Here's how the part is built. I have some questions about the finished solid (model axes, mm). A direction names the side the tool comes from. Round coordinates to 2 decimals unless told otherwise and drop trailing zeros. Loops run counter-clockwise (first coordinate to the right, second up) from the corner with the lowest first, then second, coordinate; pieces in that order, holes last. Notation, with made-up numbers: M 75.5,36.25 L 88.5,36.25 A14 cw 88.5,61.25 Z; hole C -7.75,49 d5. An arc over 180 degrees is marked long. Answer as CSV lines item,"result".
```python
from build123d import *

# Parameters (mm, degrees)
ESQUISSE1_R             = 15
BOSS_EXTRU_1_DEPTH      = 10
ESQUISSE5_R             = 6.75
ESQUISSE5_R_2           = 172
ENL_V_MAT_EXTRU_1_DEPTH = 10
CONG_1_R                = 40
ENL_V_MAT_EXTRU_2_DEPTH = 10


with BuildPart() as part:
    # Esquisse1 → Boss.-Extru.1 (new body)
    with BuildSketch(Plane(origin=(0, 0, 0), x_dir=(0, 0, -1), z_dir=(1, 0, 0))):
        Polygon((540, 0), (540, 340), (195, 340), (0, 180), (0, 0), (0, -100), (540, -100), align=None)
        with Locations((490, 300)):
            Circle(ESQUISSE1_R, mode=Mode.SUBTRACT)
        with Locations((50, 160)):
            Circle(ESQUISSE1_R, mode=Mode.SUBTRACT)
    extrude(amount=BOSS_EXTRU_1_DEPTH)

    # Esquisse5 → Enlèv. mat.-Extru.1 (cut)
    with BuildSketch(Plane.ZY):
        with Locations((-270, 325)):
            Circle(ESQUISSE5_R)
        with Locations((-217.389629624, 317.768871033)):
            Circle(ESQUISSE5_R)
        with Locations((-270, 130)):
            Circle(ESQUISSE5_R_2)
        with Locations((-168.681129743, 296.611783887)):
            Circle(ESQUISSE5_R)
        with Locations((-127.486986966, 263.097862928)):
            Circle(ESQUISSE5_R)
        with Locations((-96.862382412, 219.712682358)):
            Circle(ESQUISSE5_R)
        with Locations((-79.078602902, 169.673922545)):
            Circle(ESQUISSE5_R)
        with Locations((-75.454590008, 116.692729394)):
            Circle(ESQUISSE5_R)
        with Locations((-86.259120187, 64.698475627)):
            Circle(ESQUISSE5_R)
        with Locations((-110.690870863, 17.547337188)):
            Circle(ESQUISSE5_R)
        with Locations((-146.937850856, -21.263701687)):
            Circle(ESQUISSE5_R)
        with Locations((-192.31178748, -48.856203794)):
            Circle(ESQUISSE5_R)
        with Locations((-243.447503426, -63.183759477)):
            Circle(ESQUISSE5_R)
        with Locations((-296.552496574, -63.183759477)):
            Circle(ESQUISSE5_R)
        with Locations((-347.68821252, -48.856203794)):
            Circle(ESQUISSE5_R)
        with Locations((-393.062149144, -21.263701687)):
            Circle(ESQUISSE5_R)
        with Locations((-429.309129137, 17.547337188)):
            Circle(ESQUISSE5_R)
        with Locations((-453.740879813, 64.698475627)):
            Circle(ESQUISSE5_R)
        with Locations((-464.545409992, 116.692729394)):
            Circle(ESQUISSE5_R)
        with Locations((-460.921397098, 169.673922545)):
            Circle(ESQUISSE5_R)
        with Locations((-443.137617588, 219.712682358)):
            Circle(ESQUISSE5_R)
        with Locations((-412.513013034, 263.097862928)):
            Circle(ESQUISSE5_R)
        with Locations((-371.318870257, 296.611783887)):
            Circle(ESQUISSE5_R)
        with Locations((-322.610370376, 317.768871033)):
            Circle(ESQUISSE5_R)
        Polygon((-397.670371572, -100), (-142.329628428, -100), (0, 108.948461295), (0, -195.189428583), (-540, -195.189428583), (-540, 108.948461295), align=None)
    extrude(amount=-ENL_V_MAT_EXTRU_1_DEPTH, mode=Mode.SUBTRACT)

    # Congé1
    cong_1_edges = [part.edges().sort_by_distance(p)[0] for p in [
        (5, 180, 0),
        (5, 340, -195),
        (5, 340, -540),
    ]]
    fillet(cong_1_edges, radius=CONG_1_R)

    # Esquisse6 → Enlèv. mat.-Extru.2 (cut)
    with BuildSketch(Plane(origin=(10, 0, 0), x_dir=(0, 0, -1), z_dir=(1, 0, 0))):
        Polygon((540, -146.209782651), (540, 126.711345971), (525.303280223, 105.135676749), (533.568042486, 99.505960528), (488.530312716, 33.387862422), (480.265550453, 39.017578643), (452.116969346, -2.306232673), (460.381731609, -7.935948894), (415.344001839, -74.054047), (407.079239575, -68.424330778), (392.382519799, -90), (375, -90), (375, -100), (295, -100), (295, -90), (245, -90), (245, -100), (165, -100), (165, -90), (147.617480201, -90), (132.920760425, -68.424330778), (124.655998161, -74.054047), (79.618268391, -7.935948894), (87.883030654, -2.306232673), (59.734449547, 39.017578643), (51.469687284, 33.387862422), (6.431957514, 99.505960528), (14.696719777, 105.135676749), (0, 126.711345971), (0, -146.209782651), align=None)
    extrude(amount=-ENL_V_MAT_EXTRU_2_DEPTH, mode=Mode.SUBTRACT)


solid = part.part
```
1. I want a section at A-A, the plane z = -270. Please give me the cut outline in (x, y), and give its area (3 significant figures).
Evaluation:
outline,"M 0,-90 L 10,-90 L 10,-42 L 0,-42 Z; M 0,302 L 10,302 L 10,318.25 L 0,318.25 Z; M 0,331.75 L 10,331.75 L 10,340 L 0,340 Z"
area,"725 mm²"
2. For P1, Ø15.5, axis at y = 325, z = -270, coming from the -X side; P2, Ø5, axis at x = 3, z = -275.5, coming from the -Y side; P3, Ø1.5, axis at x = 9, y = -46.5, coming from the +Z side; P4, Ø2, axis at x = 7, y = 80, coming from the -Z side, each with a flat end and sliding along its axis, tell me the tip position at first contact or that it passes through.
Evaluation:
P1,"stops at x = 0"
P2,"stops at y = -90"
P3,"stops at z = -105.38"
P4,"stops at z = -520.96"
3. Which directions (+Z, -Z, +X, -X, +Y, -Y) give clear straight access to the entire face, cutting with the end or side of a thin tool? Please do faces 1 (the flat face through (5.07, 116.07, -532.75)), 2 (the flat face through (5.07, 115.772, -7.451)), 3 (the flat face through (5.07, -79.36, -140.37)).
Evaluation:
face 1,"-Z, +X, -X"
face 2,"+Z, +X, -X"
face 3,"+X, -X, -Y"
4. If I drill on line 1 (Y direction, x = 3, z = -270); line 2 (Y direction, x = 7.5, z = -246.5); line 3 (Z direction, x = 3, y = 260), over which ranges is the centre line in solid material (lowest first)? Write a range as [from, to].
Evaluation:
line 1,"y = [-90, -42], [302, 318.25], [331.75, 340]"
line 2,"y = [-90, -69.2], [-57.16, -40.39], [300.39, 340]"
line 3,"z = [-540, -418.51], [-406.52, -382.62], [-157.38, -133.48], [-121.49, -97.5]"
5. I want a section at B-B, the plane x = 3.25. Count the separate pieces of the cut face and the enclosed holes in it, and give its area (3 significant figures).
Evaluation:
separate pieces,"1"
enclosed holes,"26"
area,"91,300 mm²"
